Can you work these out from the model? Positions are in its coordinate system, mm. Round coordinates to 2 decimals unless told otherwise and drop trailing zeros. Write each loop counter-clockwise with the first axis right and the second up, starting at its lowest first coordinate (ties: lowest second). Pieces come first, ordered by that corner, then holes. Notation, with made-up numbers: (13.25, 27) -> (54.25, 27) arc R7 ccw to (54.25, 35) -> close; hole circle Ø1 at (35, 0). An arc over 180 degrees is marked (long way). Use CSV: the item, a comma, the result in double quotes.
```python
from build123d import *

# Parameters (mm, degrees)
FILLET_R = 3


with BuildPart() as cono:
    # Cone → Cone (revolve)
    with BuildSketch(Plane.XZ):
        Polygon((0, 0), (30, 17), (0, 17), align=None)
    revolve(axis=Axis((0, 0, 0), (0, 0, 1)))


with BuildPart() as fillet_body:
    # Cone001 → Cone001 (revolve)
    with BuildSketch(Plane(origin=(0, 0, 15), x_dir=(1, 0, 0), z_dir=(0, -1, 0))):
        Polygon((0, 0), (7, 0), (4, 15), (0, 15), align=None)
    revolve(axis=Axis((0, 0, 15), (0, 0, 1)))

    # Fusion: union Cono
    add(cono.part)

    # Fillet
    fillet_edges = [fillet_body.edges().sort_by_distance(p)[0] for p in [
        (-4, 0, 30),
    ]]
    fillet(fillet_edges, radius=FILLET_R)


solid = fillet_body.part
```
Q1. Will these pins go through, and if not, where does the flat tip stop? P1, Ø3, axis at x = -8, z = 15, coming from the +Y side; P2, Ø8, axis at x = 8, y = -19, coming from the -Z side; P3, Ø10, axis at y = 7.5, z = 25.5, coming from the -X side.
Resolved:
P1,"stops at y = 28.03"
P2,"stops at z = 9.42"
P3,"stops at x = -4.43"
Q2. Please list where these lines run through material, in increasing order: probe 1 along X at (y, z) = (-2, 15.5); probe 2 along Z at (x, y) = (-17.5, -12); probe 3 along Z at (x, y) = (-25.5, -8.5).
Resolved:
probe 1,"x = -27.28 to 27.28"
probe 2,"z = 12.02 to 17"
probe 3,"z = 15.23 to 17"
Q3. Suppose I cut it at A-A (z = 19). Write out the boundary of the cut face in (x, y), and give its area (3 significant figures).
Resolved:
outline,"circle Ø12.4 at (0, 0)"
area,"121 mm^2"
Q4. Suppose I cut it at B-B (z = 4.25). Write out the boundary of the cut face in (x, y).
Resolved:
outline,"circle Ø15 at (0, 0)"
